Model file for the job. Use its own axes, mm. A direction names the side the tool comes from. Coordinates: 2 decimals unless noted, no trailing zeros. Loops run counter-clockwise (first coordinate to the right, second up) from the corner with the lowest first, then second, coordinate; pieces in that order, holes last.
from build123d import *

# Parameters (mm, degrees)
F0_W        = 94.5233479142
F0_H        = 71.4051574469
F1_DEPTH    = 35.56
F2_R        = 25.4
F3_DEPTH    = 35.56
F4_SIZE2    = 15.24
F4_SIZE     = 10.16
F5_DEPTH    = 7.62
F7_DEPTH    = 71.4051658
F8_DEPTH    = 25.4
F9_T4_DEPTH = 203.3902674307
F9_S5_R     = 7.295449901
F9_T6_DEPTH = 104
F10_W       = 71.4051574469
F10_H       = 12.0417065918
F11_DEPTH   = 88.9
F12_W       = 19.05
F12_H       = 21.2708730352
F13_DEPTH   = 88.9
F14_W       = 19.05
F14_H       = 21.2708730352
F15_DEPTH   = 88.9
F16_R       = 5.08
F17_W       = 97.8622660041
F17_H       = 11.2377274781
F18_DEPTH   = 12.7
F19_R       = 7.62
F20_R       = 2.032
F21_W       = 212.6409783959
F21_H       = 67.3823393881
F22_DEPTH   = 8.89
F23_W       = 78.3353857696
F23_H       = 65.2360282838
F24_DEPTH   = 24.384


# Not quite as in the source:
# - a fillet or chamfer that OpenCascade refuses, or shapes differently, is made with other operations: its cross-section is extruded or revolved along the edge and cut away or added


with BuildPart() as f1:
    # F0 (on Top) → F1 (new body)
    with BuildSketch(Plane.XY):
        with Locations((0.5442798138, -0.0245943666)):
            Rectangle(F0_W, F0_H)
    extrude(amount=F1_DEPTH)

    # F2 (on Top) → F3 (cut)
    with BuildSketch(Plane.XY):
        Circle(F2_R)
    extrude(amount=F3_DEPTH, mode=Mode.SUBTRACT)

    # F4
    f4_edges = [f1.edges().sort_by_distance(p)[0] for p in [
        (47.805954, -0.024594, 35.56),
    ]]
    f4_side = f1.faces().sort_by_distance((47.805954, -0.024594, 17.78))[0]
    chamfer(f4_edges, length=F4_SIZE, length2=F4_SIZE2, reference=f4_side)

    # F5 (add): a face of the model
    f5_faces = [f1.faces().sort_by_distance(p)[0] for p in [
        (47.8059537709, -0.0245943666, 12.7),
    ]]
    extrude(f5_faces, amount=F5_DEPTH)

    # F6 (on face) → F7 (join)
    with BuildSketch(Plane(origin=(0, 35.6779843569, 0), x_dir=(-1, 0, 0), z_dir=(0, 1, 0))):
        with BuildLine():
            Line((-55.4259537709, 25.4), (-47.8059537709, 25.4))
            ThreePointArc((-47.8059537709, 25.4), (-51.6159537709, 26.473915584), (-55.4259537709, 25.4))
        make_face()
    extrude(amount=-F7_DEPTH)

    # F8 (add): a face of the model
    f8_faces = [f1.faces().sort_by_distance(p)[0] for p in [
        (55.4259537709, -0.0245943666, 12.7),
    ]]
    extrude(f8_faces, amount=F8_DEPTH)

    # F9: chamfer of 5.08 x 25.4 on 1 edges, made by hand


with BuildPart() as f9_tool2:
    # F9_s3 → F9_t4 (new body)
    with BuildSketch(Plane.XZ.offset(101.7197280819)):
        Polygon((55.4259537709, 25.4), (80.8259537709, 20.32), (80.8259537709, 25.4), align=None)
    extrude(amount=-F9_T4_DEPTH)

    # F9_s5 → F9_t6 (cut, symmetric)
    with BuildSketch(Plane.XZ):
        with Locations((51.6159537709, 19.178465683)):
            Circle(F9_S5_R)
    extrude(amount=F9_T6_DEPTH, both=True, mode=Mode.SUBTRACT)


with BuildPart() as f1_1:
    add(f1.part)

    # F9_t1: cut F9_tool2
    add(f9_tool2.part, mode=Mode.SUBTRACT)

    # F10 (on face) → F11 (join)
    with BuildSketch(Plane(origin=(-46.7173941433, 0, 0), x_dir=(0, -1, 0), z_dir=(-1, 0, 0))):
        with Locations((0.0245943666, 6.0208532959)):
            Rectangle(F10_W, F10_H)
    extrude(amount=F11_DEPTH)

    # F12 (on face) → F13 (join)
    with BuildSketch(Plane(origin=(-46.7173941433, 0, 0), x_dir=(0, -1, 0), z_dir=(-1, 0, 0))):
        with Locations((-19.7377734572, 22.6771431095)):
            Rectangle(F12_W, F12_H)
    extrude(amount=F13_DEPTH)

    # F14 (on face) → F15 (join)
    with BuildSketch(Plane(origin=(-46.7173941433, 0, 0), x_dir=(0, -1, 0), z_dir=(-1, 0, 0))):
        with Locations((18.7768059537, 22.6771431095)):
            Rectangle(F14_W, F14_H)
    extrude(amount=F15_DEPTH)

    # F16
    f16_edges = [f1_1.edges().sort_by_distance(p)[0] for p in [
        (-91.167394, 29.262773, 33.31258),
        (-91.167394, 10.212773, 33.31258),
        (-91.167394, -9.251806, 33.31258),
        (-91.167394, -28.301806, 33.31258),
        (-135.617394, 19.737773, 33.31258),
        (-135.617394, -18.776806, 33.31258),
    ]]
    fillet(f16_edges, radius=F16_R)

    # F17 (on face) → F18 (join)
    with BuildSketch(Plane(origin=(0, 35.6779843569, 0), x_dir=(-1, 0, 0), z_dir=(0, 1, 0))):
        with Locations((-2.2137388587, 17.6605703309)):
            Rectangle(F17_W, F17_H)
    extrude(amount=F18_DEPTH)

    # F19
    f19_edges = [f1_1.edges().sort_by_distance(p)[0] for p in [
        (51.144872, 48.377984, 17.66057),
    ]]
    fillet(f19_edges, radius=F19_R)

    # F20
    f20_edges = [f1_1.edges().sort_by_distance(p)[0] for p in [
        (48.913026, 46.146138, 23.279434),
        (51.144872, 38.217984, 23.279434),
        (-1.596261, 48.377984, 23.279434),
        (51.144872, 38.217984, 12.041707),
        (48.913026, 46.146138, 12.041707),
        (-1.596261, 48.377984, 12.041707),
    ]]
    fillet(f20_edges, radius=F20_R)

    # F21 (on face) → F22 (cut, symmetric)
    with BuildSketch(Plane(origin=(0, 0, 0), x_dir=(1, 0, 0), z_dir=(0, 0, -1))):
        with Locations((-27.7419649065, 0.2171527594)):
            Rectangle(F21_W, F21_H)
    extrude(amount=F22_DEPTH, both=True, mode=Mode.SUBTRACT)

    # F23 (on face) → F24 (cut)
    with BuildSketch(Plane(origin=(0, 0, 8.89), x_dir=(1, 0, 0), z_dir=(0, 0, -1))):
        with Locations((-5.8767069131, 1.2903083116)):
            Rectangle(F23_W, F23_H)
    extrude(amount=-F24_DEPTH, mode=Mode.SUBTRACT)


solid = f1_1.part
Q1. Mould opens along X. For faces 1 (the cylindrical face through (51.56, 0.475, 26.474)), 2 (the flat face through (-88, 20, 33.313)), 3 (the cylindrical face through (-134.73, 19.6, 31.1)) say: +X half, -X half, draft (parallel to the pull), parting line (faces both ways), or undercut.
Answers:
face 1: undercut
face 2: draft
face 3: -X half
Q2. Slice it at C-C (x = -63.5). List the corners of the cut face in (y, z), and give its area (3 significant figures).
Answers:
outline: (-35.73, 0) - (-33.91, 0) - (-33.91, 8.89) - (33.47, 8.89) - (33.47, 0) - (35.68, 0) - (35.68, 12.04) - (29.26, 12.04) - (29.26, 28.23) arc R5.08 ccw to (24.18, 33.31) - (15.29, 33.31) arc R5.08 ccw to (10.21, 28.23) - (10.21, 12.04) - (-9.25, 12.04) - (-9.25, 28.23) arc R5.08 ccw to (-14.33, 33.31) - (-23.22, 33.31) arc R5.08 ccw to (-28.3, 28.23) - (-28.3, 12.04) - (-35.73, 12.04) - close
area: 1,050 mm2
Q3. Flat gauge pins, fed straight in: P1, Ø5.5, axis at x = -7.5, y = 39.5, coming from the +Z side; P2, Ø21.5, axis at x = -86.5, y = 2.5, coming from the +Z side; P3, Ø5, axis at x = -87, z = 18, coming from the -Y side. Where does each tip first touch, or does it go through?
Answers:
P1: stops at z = 23.28
P2: stops at z = 32.88
P3: stops at y = -28.3
Q4. Which spindle directions (+Z, -Z, +X, -X, +Y, -Y) get a long thin tool onto all of the face, cutting with end or side? Do faces 4 (the flat face through (2, 41, 23.279)), 5 (the flat face through (-91, -9.252, 20)), 6 (the flat face through (-6, -33.908, 13)), 7 (the flat face through (-88, -19, 33.313)). Say none if no direction does.
Answers:
face 4: +Z, +X, -X, +Y
face 5: +Z, -X
face 6: -Z
face 7: +Z, -X, +Y, -Y
Q5. Slice it at D-D (y = -19). List the corners of the cut face in (x, z).
Answers:
outline: (-135.62, 0) - (-134.06, 0) - (-134.06, 8.89) - (-45.04, 8.89) - (-45.04, 33.27) - (-16.86, 33.27) - (-16.86, 35.56) - (-46.72, 35.56) - (-46.72, 33.31) - (-130.54, 33.31) arc R5.08 ccw to (-135.62, 28.23) - close; (16.86, 33.27) - (33.29, 33.27) - (33.29, 8.89) - (78.58, 8.89) - (78.58, 0) - (80.83, 0) - (80.83, 20.32) - (55.43, 25.4) arc R7.3 ccw to (47.81, 25.4) - (32.57, 35.56) - (16.86, 35.56) - close
Q6. Slice it at A-A (x = 0). List the corners of the cut face in (y, z).
Answers:
outline: (-35.73, 0) - (-33.91, 0) - (-33.91, 33.27) - (-25.4, 33.27) - (-25.4, 35.56) - (-35.73, 35.56) - close; (25.4, 33.27) - (31.33, 33.27) - (31.33, 8.89) - (33.47, 8.89) - (33.47, 0) - (35.68, 0) - (35.68, 12.04) - (46.35, 12.04) arc R2.03 ccw to (48.38, 14.07) - (48.38, 21.25) arc R2.03 ccw to (46.35, 23.28) - (35.68, 23.28) - (35.68, 35.56) - (25.4, 35.56) - close
Q7. Slice it at B-B (y = 0). List the corners of the cut face in (x, z).
Answers:
outline: (-135.62, 0) - (-134.06, 0) - (-134.06, 8.89) - (-45.04, 8.89) - (-45.04, 33.27) - (-25.4, 33.27) - (-25.4, 35.56) - (-46.72, 35.56) - (-46.72, 12.04) - (-135.62, 12.04) - close; (25.4, 33.27) - (33.29, 33.27) - (33.29, 8.89) - (78.58, 8.89) - (78.58, 0) - (80.83, 0) - (80.83, 20.32) - (55.43, 25.4) arc R7.3 ccw to (47.81, 25.4) - (32.57, 35.56) - (25.4, 35.56) - close
Q8. Drill centre lines: line 1 (X direction, y = 27, z = 4.5); line 2 (Y direction, x = 49, z = 7.5); line 3 (X direction, y = 30.5, z = 14). Where is each one in solid material? Low to high.
Answers:
line 1: x = -135.62 to -134.06, 78.58 to 80.83
line 2: y = -35.73 to -33.91, 33.47 to 35.68
line 3: x = -46.72 to -45.04, 33.29 to 80.83
